Read the model definition and answer for the solid it produces. Units are mm, in the model's axes. Coordinates: 2 decimals unless noted, no trailing zeros. Write each loop counter-clockwise with the first axis right and the second up, starting at its lowest first coordinate (ties: lowest second). Pieces come first, ordered by that corner, then holes. Notation, with made-up numbers: (12.5, 35) - (60.5, 35) arc R12 cw to (60.5, 57) - close; hole circle Ø2 at (80.25, 16.5). An arc over 180 degrees is marked (long way). Return JSON: item names as keys, results as strings.
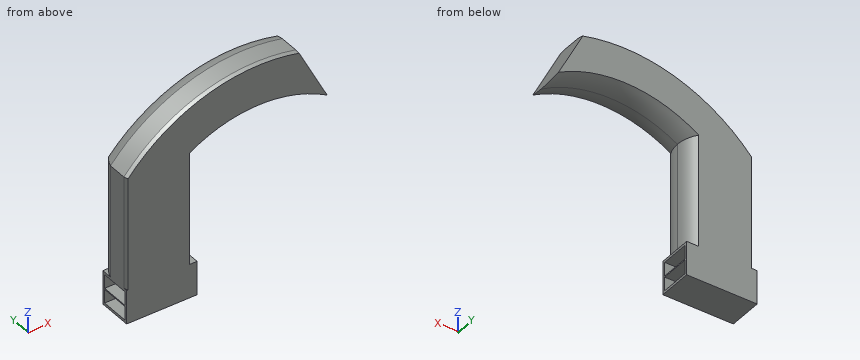
```python
from build123d import *

# Parameters (mm, degrees)
F0_W     = 50
F0_H     = 24
F1_DEPTH = 24
F3_W     = 20.4
F3_H     = 9.8
F4_DEPTH = 50.001
F5_DEPTH = 80
F7_ANGLE = 62.6704880326


with BuildPart() as f1:
    # F0 (on Front) → F1 (new body)
    with BuildSketch(Plane.XZ):
        with Locations((-68.9176678658, 12)):
            Rectangle(F0_W, F0_H)
    extrude(amount=F1_DEPTH)

    # F3 (on face) → F4 (cut, through all)
    with BuildSketch(Plane(origin=(-93.9176678658, 0, 0), x_dir=(0, -1, 0), z_dir=(-1, 0, 0))):
        with Locations((12, 6.7)):
            Rectangle(F3_W, F3_H)
        with Locations((12, 17.3)):
            Rectangle(F3_W, F3_H)
    extrude(amount=-F4_DEPTH, mode=Mode.SUBTRACT)

    # F2 (on face) → F5 (join)
    with BuildSketch(Plane.XY.offset(24)):
        with BuildLine():
            ThreePointArc((-49.4927692396, -24), (-47.9986026074, -19.3399762696), (-47.4933667129, -14.4724212587))
            ThreePointArc((-47.4933667129, -14.4724212587), (-48.7602054242, -6.8275726586), (-52.425289602, 0))
            Line((-52.425289602, 0), (-89.9617876104, 0))
            ThreePointArc((-89.9617876104, 0), (-92.2976878441, -3.6875692563), (-93.9176678658, -7.7409951716))
            Line((-93.9176678658, -7.7409951716), (-93.9176678658, -21.2038473458))
            ThreePointArc((-93.9176678658, -21.2038473458), (-93.4499426711, -22.6180106094), (-92.8943079727, -24))
            Line((-92.8943079727, -24), (-49.4927692396, -24))
        make_face()
    extrude(amount=F5_DEPTH)

    # F6 (on face) → F7 (revolve)
    with BuildSketch(Plane.XY.offset(104)):
        with BuildLine():
            ThreePointArc((-49.4927692396, -24), (-47.9986026074, -19.3399762696), (-47.4933667129, -14.4724212587))
            ThreePointArc((-47.4933667129, -14.4724212587), (-48.7602054242, -6.8275726586), (-52.425289602, 0))
            Line((-52.425289602, 0), (-89.9617876104, 0))
            ThreePointArc((-89.9617876104, 0), (-92.2976878441, -3.6875692563), (-93.9176678658, -7.7409951716))
            Line((-93.9176678658, -7.7409951716), (-93.9176678658, -21.2038473458))
            ThreePointArc((-93.9176678658, -21.2038473458), (-93.4499426711, -22.6180106094), (-92.8943079727, -24))
            Line((-92.8943079727, -24), (-49.4927692396, -24))
        make_face()
    revolve(axis=Axis((0, 2.9759369791, 24), (0, 1, 0)), revolution_arc=F7_ANGLE)


solid = f1.part
```
(1) A cutting plane is placed at A-A (z = 37). Determine the outline of the cut face in (x, y), and give its area (3 significant figures).
Answer:
{"outline": "(-93.92, -21.2) arc R23.7 ccw to (-92.89, -24) - (-49.49, -24) arc R23.7 ccw to (-52.43, 0) - (-89.96, 0) arc R23.7 ccw to (-93.92, -7.74) - close", "area": "1,070 mm²"}
(2) Flat-ended cylindrical pins translate along their axes: P1, Ø1, axis at x = -42, y = -20.5, coming from the +Z side; P2, Ø3, axis at x = -28, y = -12.5, coming from the +Z side; P3, Ø10, axis at x = -68.5, y = -9, coming from the +Z side; P4, Ø6, axis at y = -14, z = 19, coming from the +X side. Find the tip coordinate at first contact, or state that the pin passes through.
Answer:
{"P1": "z = 140.18", "P2": "z = 144.49", "P3": "z = 129.77", "P4": "through"}
(3) A cutting plane is placed at B-B (x = -72). State how many separate pieces and enclosed holes the cut face has, and give its area (3 significant figures).
Answer:
{"separate pieces": "1", "enclosed holes": "2", "area": "2,570 mm²"}
(4) Straight lines are drawn through the part: line 1 (Z direction, x = -45, y = -4) (3 decimals); line 2 (Z direction, x = -84, y = -21.75); line 3 (X direction, y = -20, z = 106). For each, find the intervals that lie inside material, in ascending order. Write a range as from..to.
Answer:
{"line 1": "0..1.8, 11.6..12.4, 22.2..24, 106.875..137.679", "line 2": "0..1.8, 11.6..12.4, 22.2..114.18", "line 3": "-92.18..-44.66, 44.66..47.67"}
